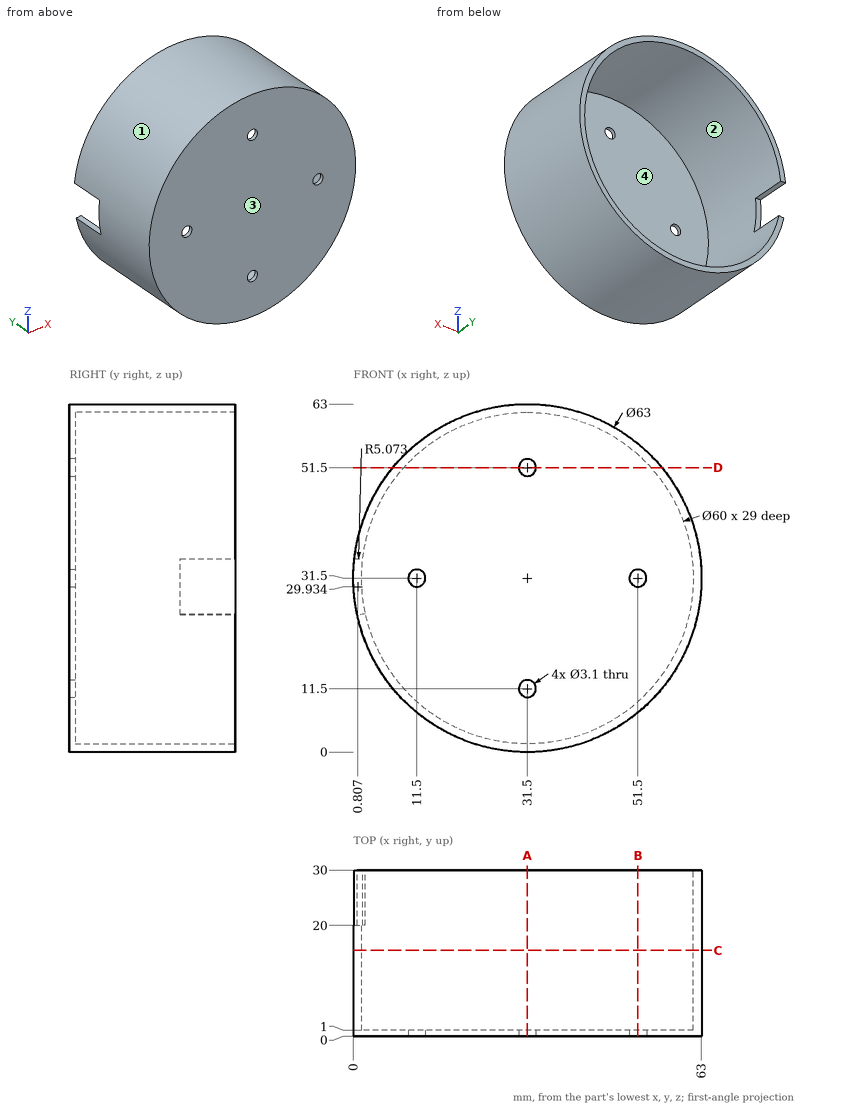
Job drawing, mm, ordinate dimensions from the low corner. One solid piece. Round coordinates to 2 decimals unless told otherwise and drop trailing zeros. Write each loop counter-clockwise with the first axis right and the second up, starting at its lowest first coordinate (ties: lowest second). Pieces come first, ordered by that corner, then holes.
1) Drill centre lines: probe 1 along X at (y, z) = (0.5, 31.5); probe 2 along Y at (x, z) = (12.5, 53.5); probe 3 along X at (y, z) = (6.75, 55.5). Where is each one in solid material? Low to high.
2) Band-saw the part on A-A, the plane x = 31.5. List the corners of the cut face in (y, z).
3) Band-saw the part on D-D, the plane z = 51.5. List the corners of the cut face in (x, y).
4) Band-saw the part on B-B, the plane x = 51.5. List the corners of the cut face in (y, z), and give its area (3 significant figures).
5) Pin check, flat tips, straight feed: pin 1 (5 mm diameter, centred on y = 5.5, z = 7.5, fed in from +X); pin 2 (3 mm diameter, centred on x = 31.5, z = 11.5, fed in from +Y); pin 3 (1.5 mm diameter, centred on y = 26.5, z = 24, fed in from -X); pin 4 (10 mm diameter, centred on x = 7, z = 50.5, fed in from -Y). Stop position of each tip, or through.
6) Mould opens along X. For the marked faces 1, 2, 3 and 4 say: +X half, -X half, draft (parallel to the pull), parting line (faces both ways), or undercut.
7) Band-saw the part on C-C, the plane y = 15.5. List the corners of the cut face in (x, z), and give its area (3 significant figures).
Ans:
1. probe 1: x = 0 to 9.95, 13.05 to 49.95, 53.05 to 63
1. probe 2: y = 0 to 1
1. probe 3: x = 11.1 to 13.5, 49.5 to 51.9
2. outline: (0, 0) - (30, 0) - (30, 1.5) - (1, 1.5) - (1, 9.95) - (0, 9.95) - close; (0, 13.05) - (1, 13.05) - (1, 49.95) - (0, 49.95) - close; (0, 53.05) - (1, 53.05) - (1, 61.5) - (30, 61.5) - (30, 63) - (0, 63) - close
3. outline: (7.16, 0) - (29.95, 0) - (29.95, 1) - (9.14, 1) - (9.14, 30) - (7.16, 30) - close; (33.05, 0) - (55.84, 0) - (55.84, 30) - (53.86, 30) - (53.86, 1) - (33.05, 1) - close
4. outline: (0, 7.16) - (30, 7.16) - (30, 9.14) - (1, 9.14) - (1, 29.95) - (0, 29.95) - close; (0, 33.05) - (1, 33.05) - (1, 53.86) - (30, 53.86) - (30, 55.84) - (0, 55.84) - close
4. area: 160 mm2
5. pin 1: stops at x = 54.52
5. pin 2: passes through
5. pin 3: stops at x = 0.73
5. pin 4: stops at y = 0
6. face 1: parting line
6. face 2: undercut
6. face 3: draft
6. face 4: undercut
7. outline: circle Ø63 at (31.5, 31.5); hole circle Ø60 at (31.5, 31.5)
7. area: 290 mm2
